Source: three-view drawing plus pictorial views. Frame: mm from the lowest corner of the part. A direction names the side the tool comes from. Give positions to 0.01 mm unless a question says otherwise; leave off trailing zeros. Loops run counter-clockwise (first coordinate to the right, second up) from the corner with the lowest first, then second, coordinate; pieces in that order, holes last. Notation, with made-up numbers: M 64,73.5 L 108,73.5 A26 cw 108,104.5 Z; hole C 72,43 d3. An arc over 180 degrees is marked long. Answer as a JSON object with one key per item and string values. Group by question number.
1) Section query A-A on x = 27.5. Return loops of the section in (y, z), plus the area to 3 significant figures.
2) Section query C-C on y = 14.5. Return loops of the section in (x, z), plus the area to 3 significant figures.
3) First-contact query: P1, Ø3, axis at y = 4.5, z = 13, coming from the +X side; P2, Ø3, axis at x = 35.5, y = 5, coming from the -Z side; P3, Ø2.5, axis at y = 14.5, z = 27.5, coming from the +X side. Flat tips, straight axial feed; report the tip coordinate or a pass-through.
4) Draft query along Y for the marked faces 3, 4 and 5. Return one class per face: +Y half, -Y half, draft (parallel to the pull), parting line (faces both ways), or undercut.
5) Access query for the marked faces 1 and 2. Directions: +Z, -Z, +X, -X, +Y, -Y. A direction counts if a zero-diameter tool reaches every point of the face in a straight line with its end or side. Return the directions, or none.
6) Ray query, L1, parallel to Y at x = 33.25, z = 27.5; L2, parallel to Y at x = 15.5, z = 50.5; L3, parallel to Y at x = 18, z = 48.5. Return the intervals inside material, ascending.
7) Section query D-D on x = 36. Return loops of the section in (y, z).
8) Section query B-B on z = 27.5. Return loops of the section in (x, y), plus the area to 3 significant figures.
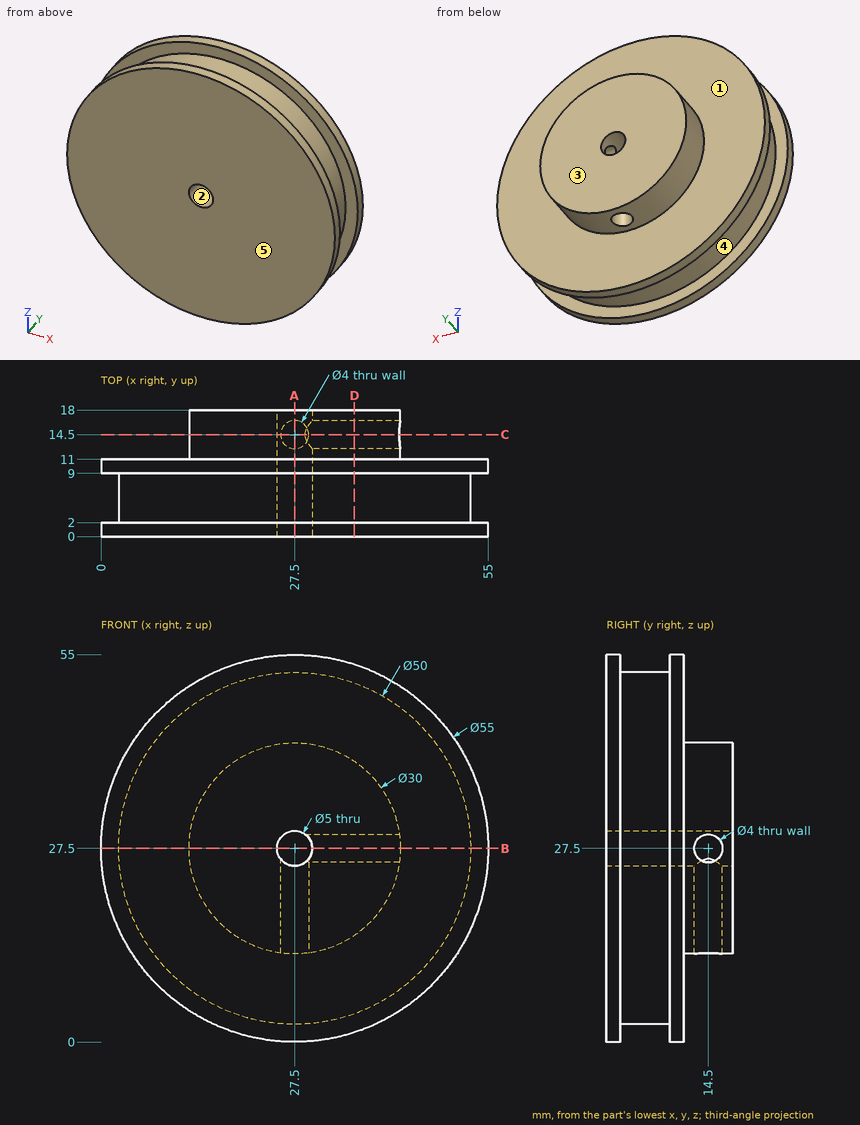
Output:
{
 "1": {"outline": "M 0,0 L 2,0 L 2,2.5 L 9,2.5 L 9,0 L 11,0 L 11,12.5 L 12.5,12.5 L 12.5,25 L 0,25 Z; M 0,30 L 18,30 L 18,42.5 L 11,42.5 L 11,55 L 9,55 L 9,52.5 L 2,52.5 L 2,55 L 0,55 Z; M 16.5,12.5 L 18,12.5 L 18,25 L 16.5,25 Z", "area": "640 mm^2"},
 "2": {"outline": "M 25.5,12.63 L 25.5,26 A2.5 cw 29,29.5 L 42.37,29.5 A15 ccw long Z; M 29.5,12.63 A15 ccw 42.37,25.5 L 29.5,25.5 Z", "area": "585 mm^2"},
 "3": {"P1": "stops at x = 48.85", "P2": "stops at z = 3.36", "P3": "stops at x = 25.33"},
 "4": {"face 3": "+Y half", "face 4": "undercut", "face 5": "-Y half"},
 "5": {"face 1": "+Y", "face 2": "+Y, -Y"},
 "6": {"L1": "y = 0 to 12.5, 16.5 to 18", "L2": "y = 0 to 2, 9 to 11", "L3": "y = 0 to 11"},
 "7": {"outline": "M 0,1.35 L 2,1.35 L 2,3.99 L 9,3.99 L 9,1.35 L 11,1.35 L 11,15.14 L 18,15.14 L 18,39.86 L 11,39.86 L 11,53.65 L 9,53.65 L 9,51.01 L 2,51.01 L 2,53.65 L 0,53.65 Z; hole C 14.5,27.5 d4"},
 "8": {"outline": "M 0,0 L 25,0 L 25,18 L 12.5,18 L 12.5,11 L 0,11 L 0,9 L 2.5,9 L 2.5,2 L 0,2 Z; M 30,0 L 55,0 L 55,2 L 52.5,2 L 52.5,9 L 55,9 L 55,11 L 42.5,11 L 42.5,12.5 L 30,12.5 Z; M 30,16.5 L 42.5,16.5 L 42.5,18 L 30,18 Z", "area": "640 mm^2"}
}
